```python
from build123d import *

# Parameters (mm, degrees)
Y_KSEKLIK_EKSTR_ZYON1_DEPTH = 5
IZIM2_R                     = 1.5
KES_EKSTR_ZYON1_DEPTH       = 15
KES_EKSTR_ZYON2_DEPTH       = 2.5


with BuildPart() as part:
    # Çizim1 → Yükseklik-Ekstrüzyon1 (new, symmetric)
    with BuildSketch(Plane.XY):
        with BuildLine():
            Line((-41.30834423, 28.453834486), (-2.524523213, -3.102705681))
            ThreePointArc((-2.524523213, -3.102705681), (-0.805425984, -3.9180721), (1.095904798, -3.846945889))
            Line((1.095904798, -3.846945889), (15.52194925, 0.262696355))
            ThreePointArc((15.52194925, 0.262696355), (17.169826346, 1.200432935), (18.198993637, 2.792809619))
            Line((18.198993637, 2.792809619), (21.476713619, 12.240378181))
            ThreePointArc((21.476713619, 12.240378181), (19.014364959, 17.318962653), (13.935780486, 14.856613993))
            Line((13.935780486, 14.856613993), (11.337646141, 7.367855803))
            Line((11.337646141, 7.367855803), (0.900459327, 4.382653193))
            Line((0.900459327, 4.382653193), (-36.257215818, 34.657550675))
            ThreePointArc((-36.257215818, 34.657550675), (-41.885679286, 34.082104516), (-41.30834423, 28.453834486))
        make_face()
    extrude(amount=Y_KSEKLIK_EKSTR_ZYON1_DEPTH, both=True)

    # Çizim2 → Kes-Ekstrüzyon1 (cut)
    with BuildSketch(Plane.XY.offset(5)):
        with Locations((17.706247053, 13.548496087)):
            Circle(IZIM2_R)
        Circle(IZIM2_R)
    extrude(amount=-KES_EKSTR_ZYON1_DEPTH, mode=Mode.SUBTRACT)

    # Çizim3 → Kes-Ekstrüzyon2 (cut, symmetric)
    with BuildSketch(Plane.XY):
        with BuildLine():
            Line((12.739401972, 11.408220568), (20.280335105, 8.791984755))
            Line((20.280335105, 8.791984755), (21.476713619, 12.240378181))
            ThreePointArc((21.476713619, 12.240378181), (19.014364959, 17.318962653), (13.935780486, 14.856613993))
            Line((13.935780486, 14.856613993), (12.739401972, 11.408220568))
        make_face()
    extrude(amount=KES_EKSTR_ZYON2_DEPTH, both=True, mode=Mode.SUBTRACT)


solid = part.part
```
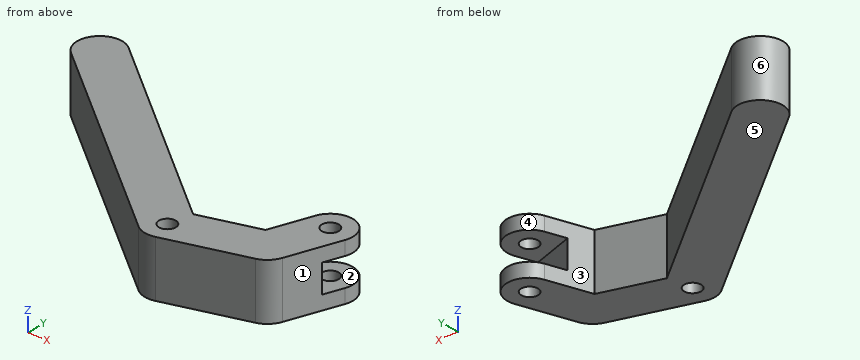
Could you check a few things on this model? Use its own coordinates, in mm. Face numbers are marked on the shaded views. A direction names the side the tool comes from. Round coordinates to 2 decimals unless told otherwise and drop trailing zeros. Loops run counter-clockwise (first coordinate to the right, second up) from the corner with the lowest first, then second, coordinate; pieces in that order, holes last. Notation, with made-up numbers: (-18.5, 17.25) - (16.5, 17.25) arc R26 ccw to (16.5, 31.25) - close; hole circle Ø8 at (26.5, 37.5). An arc over 180 degrees is marked (long way). Answer in a Markdown table with one row per item. Add a question column.
(1) If we section it at C-C (z = 3.5): Please give me the cut outline in (x, y).
(2) If we section it at D-D (x = -10.5): Please give me the cut outline in (y, z), plus the area to 3 significant figures.
(3) I need wall thicknesses on line 1 along Z through (x, y) = (15.5, 16.5); line 2 along X through (y, z) = (13, 4); line 3 along Y through (x, z) = (0, -1.5). Which ranges of each line are inside material? Lowest first, please.
(4) If we mould it in two halves opening along X, with no side actions, what happens to the marked faces 4, 5 and 6? For each: pulls with the +X half, pulls with the -X half, needs draft (parallel to the pull), parting line crosses it, or undercut.
(5) For the marked faces 1, 2 and 3, which set-ups out of +Z, -Z, +X, -X, +Y, -Y let a thin tool reach every point of the face, with its end or its side?
(6) If we section it at B-B (x = 0): Please give me the cut outline in (y, z), plus the area to 3 significant figures.
(7) If we section it at A-A (z = -0.5): Please give me the cut outline in (x, y).
(8) I'm going to push flat-ended pins straight in: pin 1 (4 mm diameter, centred on x = -29.5, z = 1, fed in from +Y); pin 2 (1 mm diameter, centred on y = 26, z = -1, fed in from +X); pin 3 (6 mm diameter, centred on y = 0.5, z = -2, fed in from -X); pin 4 (1.8 mm diameter, centred on x = 17.71, y = 13.55, fed in from -Z). Where does each tip first touch, or does it pass through?
Model answer:
| question | item | result |
|---|---|---|
| 1 | outline | (-41.31, 28.45) - (-2.52, -3.1) arc R4 ccw to (1.1, -3.85) - (15.52, 0.26) arc R3.99 ccw to (18.2, 2.79) - (21.48, 12.24) arc R3.99 ccw to (13.94, 14.86) - (11.34, 7.37) - (0.9, 4.38) - (-36.26, 34.66) arc R4 ccw to start; hole circle Ø3 at (0, 0); hole circle Ø3 at (17.71, 13.55) |
| 2 | outline | (3.39, -5) - (13.67, -5) - (13.67, 5) - (3.39, 5) - close |
| 2 | area | 103 mm² |
| 3 | line 1 | z = -5 to -2.5, 2.5 to 5 |
| 3 | line 2 | x = -22.32 to -9.68, 13.29 to 16.31, 19.1 to 21.66 |
| 3 | line 3 | y = -4 to -1.5, 1.5 to 5.12 |
| 4 | face 4 | undercut |
| 4 | face 5 | needs draft |
| 4 | face 6 | parting line crosses it |
| 5 | face 1 | +Z, -Z, +X, -Y |
| 5 | face 2 | +X, +Y |
| 5 | face 3 | +Z, -Z, +Y |
| 6 | outline | (-4, -5) - (-1.5, -5) - (-1.5, 5) - (-4, 5) - close; (1.5, -5) - (5.12, -5) - (5.12, 5) - (1.5, 5) - close |
| 6 | area | 61.2 mm² |
| 7 | outline | (-41.31, 28.45) - (-2.52, -3.1) arc R4 ccw to (1.1, -3.85) - (15.52, 0.26) arc R3.99 ccw to (18.2, 2.79) - (20.28, 8.79) - (12.74, 11.41) - (11.34, 7.37) - (0.9, 4.38) - (-36.26, 34.66) arc R4 ccw to start; hole circle Ø3 at (0, 0) |
| 8 | pin 1 | stops at y = 30.78 |
| 8 | pin 2 | stops at x = -25.02 |
| 8 | pin 3 | stops at x = -10.64 |
| 8 | pin 4 | passes through |
